Autodesk Inventor part; units mm, degrees
ref_plane "YZ Plane" through (0, 0, 0) normal (1, 0, 0) x (0, 1, 0)
ref_plane "XZ Plane" through (0, 0, 0) normal (0, 1, 0) x (-1, 0, 0)
ref_plane "XY Plane" through (0, 0, 0) normal (0, 0, 1) x (1, 0, 0)
sketch "Sketch1" plane through (0, 0, 0) normal (0, 0, 1) x (1, 0, 0)
  line L0 (0, 0) -> (431.8, 0)
  line L1 (406.4, 69.85) -> (0, 69.85)
  line L2 (0, 69.85) -> (0, 0)
  line L3 (406.4, 69.85) -> (406.4, 6.35)
  line L4 (406.4, 6.35) -> (431.8, 6.35)
  line L5 (431.8, 6.35) -> (431.8, 0)
  dimension "d0" = 69.85
  dimension "d1" = 431.8
  dimension "d2" = 6.35
  dimension "d3" = 25.4
extrude "Extrusion1" add sketch "Sketch1" along normal blind 685.8
sketch "Sketch2" plane through (0, 0, 0) normal (-1, 0, 0) x (0, 0, 1)
  line L0 (0, 0) -> (685.8, 0)
  line L1 (685.8, 69.85) -> (647.7, 69.85)
  line L2 (647.7, 69.85) -> (647.7, 6.35)
  line L3 (647.7, 6.35) -> (685.8, 6.35)
  line L4 (685.8, 6.35) -> (685.8, 69.85)
  line L5 (0, 69.85) -> (38.1, 69.85)
  line L6 (38.1, 69.85) -> (38.1, 6.35)
  line L7 (38.1, 6.35) -> (0, 6.35)
  line L8 (0, 6.35) -> (0, 69.85)
  dimension "d6" = 6.35
  dimension "d7" = 38.1
extrude "Extrusion2" cut sketch "Sketch2" against normal through all
properties part number "ElectronicsVolume"
Part model, mm, in its own coordinate system. A direction names the side the tool comes from. Give positions to 0.01 mm unless a question says otherwise; leave off trailing zeros. Write each loop counter-clockwise with the first axis right and the second up, starting at its lowest first coordinate (ties: lowest second). Pieces come first, ordered by that corner, then holes. Notation, with made-up numbers: (8, 68.5) -> (15, 68.5) arc R13 ccw to (15, 83.5) -> close; hole circle Ø4 at (72, 56.5). An arc over 180 degrees is marked (long way). Put each result on its own line as item: value. Start each with the question number.
Item 1: Cut at B-B (z = 400.5). List the corners of the cut face in (x, y), then the cut area to 3 significant figures.
Item 2: Cut at C-C (y = 63). List the corners of the cut face in (x, z), then the cut area to 3 significant figures.
Item 3: Cut at A-A (x = 104.5). List the corners of the cut face in (y, z).
Item 4: Wall check: L1, parallel to Z at x = 71, y = 15; L2, parallel to X at y = 50.5, z = 446.5. Give the ranges that are in metal, low to high. Write a range as [from, to].
Item 5: Pin check, flat tips, straight feed: pin 1 Ø2 at (y, z) = (54.5, 431) entering from +X; pin 2 Ø19 at (x, y) = (242, 30) entering from -Z. Stop position of each tip, or through.
Item 6: Which spindle directions (+Z, -Z, +X, -X, +Y, -Y) get a long thin tool onto all of the face, cutting with end or side? Do faces 1 (the face through (213, 0, 338)), 2 (the face through (200, 39, 38.1)), 3 (the face through (206, 69.85, 339)), 4 (the face through (406.4, 39, 339)), 5 (the face through (200, 39, 647.7)). Say none if no direction does.
Answer list:
1. outline: (0, 0) -> (431.8, 0) -> (431.8, 6.35) -> (406.4, 6.35) -> (406.4, 69.85) -> (0, 69.85) -> close
1. area: 28,500 mm2
2. outline: (0, 38.1) -> (406.4, 38.1) -> (406.4, 647.7) -> (0, 647.7) -> close
2. area: 248,000 mm2
3. outline: (0, 0) -> (6.35, 0) -> (6.35, 38.1) -> (69.85, 38.1) -> (69.85, 647.7) -> (6.35, 647.7) -> (6.35, 685.8) -> (0, 685.8) -> close
4. L1: z = [38.1, 647.7]
4. L2: x = [0, 406.4]
5. pin 1: stops at x = 406.4
5. pin 2: stops at z = 38.1
6. face 1: +Z, -Z, +X, -X, -Y
6. face 2: -Z, +X, -X, +Y
6. face 3: +Z, -Z, +X, -X, +Y
6. face 4: +Z, -Z, +X, +Y
6. face 5: +Z, +X, -X, +Y
